Source: CAD feature listing. Evaluate the final solid. Frame: model axes, mm. Face numbers are marked on the shaded views. Give positions to 0.01 mm unless a question says otherwise; leave off trailing zeros. Loops run counter-clockwise (first coordinate to the right, second up) from the corner with the lowest first, then second, coordinate; pieces in that order, holes last.
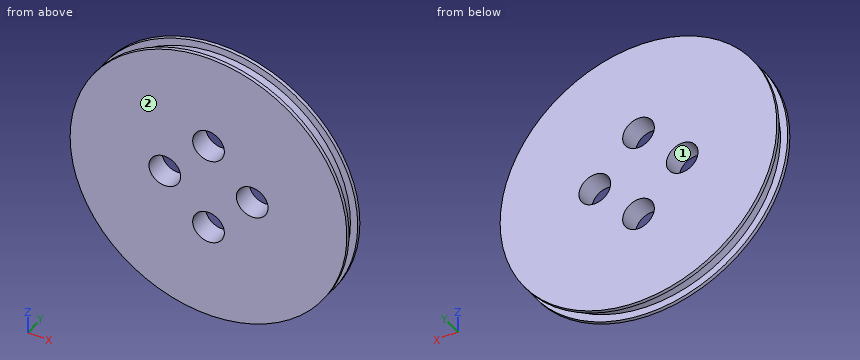
Autodesk Inventor part; units mm, degrees
ref_plane "YZ Plane" through (0, 0, 0) normal (1, 0, 0) x (0, 1, 0)
ref_plane "XZ Plane" through (0, 0, 0) normal (0, 1, 0) x (-1, 0, 0)
ref_plane "XY Plane" through (0, 0, 0) normal (0, 0, 1) x (1, 0, 0)
sketch "Sketch1" plane through (0, 0, 0) normal (0, 1, 0) x (-1, 0, 0)
  circle A0 centre (0, 0) radius 19
  dimension "d0" = 38
extrude "Extrusion1" add sketch "Sketch1" along normal blind 0.5
sketch "Sketch2" plane through (0, 0.5, 0) normal (0, 1, 0) x (1, 0, 0)
  circle A0 centre (0, 0) radius 18
  dimension "d3" = 36
extrude "Extrusion2" add sketch "Sketch2" along normal blind 2
sketch "Sketch3" plane through (0, 2.5, 0) normal (0, 1, 0) x (1, 0, 0)
  circle A0 centre (0, 0) radius 19
  dimension "d23" = 38
extrude "Extrusion3" add sketch "Sketch3" along normal blind 0.5
sketch "Sketch4" plane through (0, 3, 0) normal (0, 1, 0) x (1, 0, 0)
  circle A0 centre (0, -6) radius 2.175
  circle A1 centre (0, 6) radius 2.175
  circle A2 centre (6, 0) radius 2.175
  circle A3 centre (-6, 0) radius 2.175
  point P0 (0, 0)
  dimension "d8" = 4.35
  dimension "d9" = 6
  dimension "d10" = 4.35
  dimension "d11" = 6
  dimension "d12" = 4.35
  dimension "d13" = 6
  dimension "d14" = 4.35
  dimension "d15" = 6
hole "Hole1" at (6, 3, 0) at (0, 3, 6) at (-6, 3, 0) at (0, 3, -6) direction (0, -1, 0) diameter 4.35 end through all
properties part number "wheel"
(1) First-contact query: pin 1 (2.5 mm diameter, centred on x = -6, z = 0, fed in from +Y). Flat tip, straight axial feed; report the tip coordinate or a pass-through.
A:
pin 1: passes through
(2) Mould query, pull axis X, two halves, no side actions, for the marked faces 1 and 2. Classes: pulls with the +X half, pulls with the -X half, needs draft (parallel to the pull), parting line crosses it, or undercut.
A:
face 1: undercut
face 2: needs draft
(3) Section B-B, the plane z = 0. Return the cut outline in (x, y) (3 decimals).
A:
outline: (-19, 0) - (-8.175, 0) - (-8.175, 3) - (-19, 3) - (-19, 2.5) - (-18, 2.5) - (-18, 0.5) - (-19, 0.5) - close; (-3.825, 0) - (3.825, 0) - (3.825, 3) - (-3.825, 3) - close; (8.175, 0) - (19, 0) - (19, 0.5) - (18, 0.5) - (18, 2.5) - (19, 2.5) - (19, 3) - (8.175, 3) - close
(4) Section C-C, the plane z = 5.5. Return the cut outline in (x, y).
A:
outline: (-18.19, 0) - (-2.12, 0) - (-2.12, 3) - (-18.19, 3) - (-18.19, 2.5) - (-17.14, 2.5) - (-17.14, 0.5) - (-18.19, 0.5) - close; (2.12, 0) - (18.19, 0) - (18.19, 0.5) - (17.14, 0.5) - (17.14, 2.5) - (18.19, 2.5) - (18.19, 3) - (2.12, 3) - close
(5) Section A-A, the plane x = 0. Return the cut outline in (y, z) (3 decimals), then the cut area to 3 significant figures.
A:
outline: (0, -19) - (0.5, -19) - (0.5, -18) - (2.5, -18) - (2.5, -19) - (3, -19) - (3, -8.175) - (0, -8.175) - close; (0, -3.825) - (3, -3.825) - (3, 3.825) - (0, 3.825) - close; (0, 8.175) - (3, 8.175) - (3, 19) - (2.5, 19) - (2.5, 18) - (0.5, 18) - (0.5, 19) - (0, 19) - close
area: 83.9 mm2
(6) Ray query, line 1 along X through (y, z) = (2, 0) (3 decimals); line 2 along X through (y, z) = (2.65, 0) (3 decimals). Return the intervals inside material, ascending.
A:
line 1: x = -18 to -8.175, -3.825 to 3.825, 8.175 to 18
line 2: x = -19 to -8.175, -3.825 to 3.825, 8.175 to 19
(7) Section D-D, the plane x = -7.5. Return the cut outline in (y, z) (3 decimals).
A:
outline: (0, -17.457) - (0.5, -17.457) - (0.5, -16.363) - (2.5, -16.363) - (2.5, -17.457) - (3, -17.457) - (3, -1.575) - (0, -1.575) - close; (0, 1.575) - (3, 1.575) - (3, 17.457) - (2.5, 17.457) - (2.5, 16.363) - (0.5, 16.363) - (0.5, 17.457) - (0, 17.457) - close
